```python
from build123d import *

# Parameters (mm, degrees)
BOSS_EXTRUDE1_DEPTH  = 12.5
BOSS_EXTRUDE2_DEPTH  = 3.4
BOSS_EXTRUDE3_DEPTH  = 3.5000000000000004
SKETCH4_W            = 0.40000000000000124
SKETCH4_H            = 6.935639852470931
CUT_EXTRUDE1_DEPTH   = 15.890601062415177
CUT_EXTRUDE2_DEPTH   = 18.660124574872064
BOSS_EXTRUDE4_DEPTH  = 0.29999999999999993
SKETCH7_W            = 1.7000000000000002
SKETCH7_H            = 9.6
BOSS_EXTRUDE5_DEPTH  = 0.5000000000000003
BOSS_EXTRUDE6_DEPTH  = 0.3
CUT_EXTRUDE3_DEPTH   = 15.890601062415183
SKETCH10_W           = 1.4499999999999997
SKETCH10_H           = 1
BOSS_EXTRUDE7_DEPTH  = 0.3
BOSS_EXTRUDE8_DEPTH  = 0.3
BOSS_EXTRUDE9_START  = 0.3
BOSS_EXTRUDE9_DEPTH  = 0.3
SKETCH13_W           = 3.3000000000000003
SKETCH13_H           = 0.3
CUT_EXTRUDE4_DEPTH   = 16.455824144962317
SKETCH14_W           = 3.3
SKETCH14_H           = 0.3
CUT_EXTRUDE5_DEPTH   = 1.7
SKETCH15_W           = 3.3
SKETCH15_H           = 0.3
CUT_EXTRUDE6_DEPTH   = 18.38620142526826
CUT_EXTRUDE7_REACH   = 19.386
SKETCH16_W           = 3.3
SKETCH16_H           = 0.3
BOSS_EXTRUDE10_DEPTH = 1.14
BOSS_EXTRUDE11_DEPTH = 1.14
BOSS_EXTRUDE12_DEPTH = 1.14
BOSS_EXTRUDE13_DEPTH = 1.14
CUT_EXTRUDE8_DEPTH   = 9.1
SKETCH22_W           = 1.1399999999999995
SKETCH22_H           = 1.1400000000000003
BOSS_EXTRUDE14_DEPTH = 5.6000000000000005
SKETCH23_W           = 3.5
SKETCH23_H           = 3.4999999999999996
CUT_EXTRUDE9_DEPTH   = 9.1
SKETCH24_W           = 1.14
SKETCH24_H           = 1.1400000000000003
BOSS_EXTRUDE15_DEPTH = 5.6000000000000005
CUT_EXTRUDE10_DEPTH  = 9.1
BOSS_EXTRUDE16_DEPTH = 5.6000000000000005
SKETCH27_W           = 3.5
SKETCH27_H           = 3.4999999999999996
CUT_EXTRUDE11_DEPTH  = 9.1
SKETCH28_W           = 1.1399999999999995
SKETCH28_H           = 1.1400000000000006
BOSS_EXTRUDE17_DEPTH = 5.6000000000000005
DRAFT1_ANGLE         = -5.000000000000134
DRAFT2_ANGLE         = 39.99999999999766
CHAMFER1_SIZE        = 1.0000000000000708
CHAMFER2_SIZE        = 0.7999999999999999
FILLET1_R            = 0.3


with BuildPart() as part:
    # Sketch1 → Boss-Extrude1 (new body)
    with BuildSketch(Plane.XZ.offset(-0.3)):
        with BuildLine():
            Line((-4.8, -4.8), (1.7000000000000002, -4.8))
            Line((1.7000000000000002, -4.8), (1.7000000000000002, 4.800000000000001))
            Line((1.7000000000000002, 4.800000000000001), (-4.8, 4.8))
            Line((-4.8, 4.8), (-4.8, -2.2))
            ThreePointArc((-4.8, -2.2), (-5.2, -2.6000000000000005), (-4.8, -3.0000000000000004))
            Line((-4.8, -3.0000000000000004), (-4.8, -4.8))
        make_face()
    extrude(amount=-BOSS_EXTRUDE1_DEPTH)

    # Sketch2 → Boss-Extrude2 (add)
    with BuildSketch(Plane(origin=(1.7, 0, 0), x_dir=(0, 0, -1), z_dir=(1, 0, 0))):
        Polygon((-4.800000000000008, 12.800000000000006), (-6.200000000000001, 10.45), (-6.200000000000001, 9.627515871063899), (-4.800000000000008, 9.627515871063899), align=None)
    extrude(amount=-BOSS_EXTRUDE2_DEPTH)

    # Sketch3 → Boss-Extrude3 (add)
    with BuildSketch(Plane(origin=(1.7000000000000002, 0, 0), x_dir=(0, 0, -1), z_dir=(1, 0, 0))):
        Polygon((4.8, 0.29999999999999993), (-4.800000000000001, 0.29999999999999993), (-4.8, 12.8), (4.8, 12.8), align=None)
    extrude(amount=BOSS_EXTRUDE3_DEPTH)

    # Sketch4 → Cut-Extrude1 (cut, through all)
    with BuildSketch(Plane(origin=(0, 12.8, 0), x_dir=(-1, 0, 0), z_dir=(0, 1, 0))):
        with Locations((-5, -1.3321800737645344)):
            Rectangle(SKETCH4_W, SKETCH4_H)
    extrude(amount=-CUT_EXTRUDE1_DEPTH, mode=Mode.SUBTRACT)

    # Sketch5 → Cut-Extrude2 (cut, through all)
    with BuildSketch(Plane(origin=(0, 0, -4.8), x_dir=(-1, 0, 0), z_dir=(0, 0, -1))):
        Polygon((-3.35, 0.29999999999999993), (3.3499999999999996, 0.29999999999999993), (3.35, 0.5000000000000001), (-3.35, 0.5000000000000004), align=None)
    extrude(amount=-CUT_EXTRUDE2_DEPTH, mode=Mode.SUBTRACT)

    # Sketch6 → Boss-Extrude4 (add)
    with BuildSketch(Plane.XZ.offset(-0.3)):
        Polygon((4.8, -4.8), (3.35, -4.8), (3.35, 0.49999999999999956), (4.8, 0.5), align=None)
    extrude(amount=BOSS_EXTRUDE4_DEPTH)

    # Sketch7 → Boss-Extrude5 (add)
    with BuildSketch(Plane.XZ.offset(-0.5000000000000002)):
        Rectangle(SKETCH7_W, SKETCH7_H)
    extrude(amount=BOSS_EXTRUDE5_DEPTH)

    # Sketch8 → Boss-Extrude6 (add)
    with BuildSketch(Plane.XZ.offset(-0.3)):
        Polygon((-4.8, -4.8), (-4.8, -3.8), (-3.3499999999999996, -3.8), (-3.35, -4.8), align=None)
    extrude(amount=BOSS_EXTRUDE6_DEPTH)

    # Sketch9 → Cut-Extrude3 (cut, through all)
    with BuildSketch(Plane.XZ.offset(-0.3)):
        Polygon((5.200000000000001, 4.800000000000001), (4.8, 4.800000000000001), (4.8, 3.464360147529), (5.200000000000001, 3.4643601475289993), align=None)
    extrude(amount=-CUT_EXTRUDE3_DEPTH, mode=Mode.SUBTRACT)

    # Sketch10 → Boss-Extrude7 (add)
    with BuildSketch(Plane.XZ.offset(-0.3)):
        with Locations((4.075, 4.3)):
            Rectangle(SKETCH10_W, SKETCH10_H)
    extrude(amount=BOSS_EXTRUDE7_DEPTH)

    # Sketch11 → Boss-Extrude8 (add)
    with BuildSketch(Plane.XZ.offset(-0.3)):
        Polygon((-4.8, 4.8), (-3.3499999999999996, 4.8), (-3.35, -0.49999999999999956), (-4.8, -0.5), align=None)
    extrude(amount=BOSS_EXTRUDE8_DEPTH)

    # Sketch12 → Boss-Extrude9 (add)
    with BuildSketch(Plane.XZ.offset(-0.3).offset(BOSS_EXTRUDE9_START)):
        with BuildLine():
            Line((-4.8, -2.2), (-4.8, -3.0000000000000004))
            ThreePointArc((-4.8, -3.0000000000000004), (-5.199999999999999, -2.6000000000000005), (-4.8, -2.2))
        make_face()
    extrude(amount=-BOSS_EXTRUDE9_DEPTH)

    # Sketch13 → Cut-Extrude4 (cut, through all)
    with BuildSketch(Plane.ZY.offset(0.8500000000000001)):
        with Locations((2.15, 0.15000000000000005)):
            Rectangle(SKETCH13_W, SKETCH13_H)
    extrude(amount=-CUT_EXTRUDE4_DEPTH, mode=Mode.SUBTRACT)

    # Sketch14 → Cut-Extrude5 (cut)
    with BuildSketch(Plane.ZY.offset(0.8500000000000001)):
        with Locations((-2.15, 0.15000000000000005)):
            Rectangle(SKETCH14_W, SKETCH14_H)
    extrude(amount=-CUT_EXTRUDE5_DEPTH, mode=Mode.SUBTRACT)

    # Sketch15 → Cut-Extrude6 (cut, through all)
    with BuildSketch(Plane.ZY.offset(4.8)):
        with Locations((2.15, 0.15)):
            Rectangle(SKETCH15_W, SKETCH15_H)
    extrude(amount=-CUT_EXTRUDE6_DEPTH, mode=Mode.SUBTRACT)

    # Sketch16 → Cut-Extrude7 (cut, up to next)
    with BuildSketch(Plane(origin=(4.8, 0, 0), x_dir=(0, 0, -1), z_dir=(1, 0, 0)), mode=Mode.PRIVATE) as cut_extrude7_sk1:
        with Locations((2.15, 0.15)):
            Rectangle(SKETCH16_W, SKETCH16_H)
    cut_extrude7_tool1 = extrude(cut_extrude7_sk1.sketch, amount=-CUT_EXTRUDE7_REACH, mode=Mode.PRIVATE) & part.part
    add(cut_extrude7_tool1.solids().sort_by_distance((4.8, 0.15, -2.15))[0], mode=Mode.SUBTRACT)

    # Sketch17 → Boss-Extrude10 (add)
    with BuildSketch(Plane(origin=(1.53, 0, 0), x_dir=(0, -1, 0), z_dir=(-1, 0, 0))):
        Polygon((2.500000000000003, 2.6499999999999937), (3.5, 3.085), (3.5, 3.2500000000000004), (-0.5, 3.2500000000000004), (-0.5, 2.6500000000000004), align=None)
    extrude(amount=-BOSS_EXTRUDE10_DEPTH)

    # Sketch18 → Boss-Extrude11 (add)
    with BuildSketch(Plane(origin=(1.53, 0, 0), x_dir=(0, -1, 0), z_dir=(-1, 0, 0))):
        Polygon((3.5, -2.85), (3.4999999999999987, -2.685000000000003), (2.5000000000000004, -2.2500000000000004), (-0.5, -2.2500000000000004), (-0.5, -2.85), align=None)
    extrude(amount=-BOSS_EXTRUDE11_DEPTH)

    # Sketch19 → Boss-Extrude12 (add)
    with BuildSketch(Plane(origin=(-2.6700000000000004, 0, 0), x_dir=(0, -1, 0), z_dir=(-1, 0, 0))):
        Polygon((2.500000000000003, 2.6499999999999937), (3.5, 3.085), (3.5, 3.2500000000000004), (-0.5, 3.2500000000000004), (-0.5, 2.6500000000000004), align=None)
    extrude(amount=-BOSS_EXTRUDE12_DEPTH)

    # Sketch20 → Boss-Extrude13 (add)
    with BuildSketch(Plane(origin=(-2.6700000000000004, 0, 0), x_dir=(0, -1, 0), z_dir=(-1, 0, 0))):
        Polygon((3.5, -2.85), (3.4999999999999987, -2.685000000000003), (2.5000000000000004, -2.2500000000000004), (-0.5, -2.2500000000000004), (-0.5, -2.85), align=None)
    extrude(amount=-BOSS_EXTRUDE13_DEPTH)

    # Sketch21 → Cut-Extrude8 (cut)
    with BuildSketch(Plane(origin=(0, 12.8, 0), x_dir=(-1, 0, 0), z_dir=(0, 1, 0))):
        Polygon((0.3499999999999999, 4.05), (0.34999999999999964, 0.5500000000000002), (3.85, 0.5500000000000002), (3.85, 4.05), align=None)
    extrude(amount=-CUT_EXTRUDE8_DEPTH, mode=Mode.SUBTRACT)

    # Sketch22 → Boss-Extrude14 (add)
    with BuildSketch(Plane(origin=(0, 3.7, 0), x_dir=(-1, 0, 0), z_dir=(0, 1, 0))):
        with Locations((2.0999999999999996, 2.3)):
            Rectangle(SKETCH22_W, SKETCH22_H)
    extrude(amount=BOSS_EXTRUDE14_DEPTH)

    # Sketch23 → Cut-Extrude9 (cut)
    with BuildSketch(Plane(origin=(0, 12.8, 0), x_dir=(-1, 0, 0), z_dir=(0, 1, 0))):
        with Locations((-2.1, 2.3)):
            Rectangle(SKETCH23_W, SKETCH23_H)
    extrude(amount=-CUT_EXTRUDE9_DEPTH, mode=Mode.SUBTRACT)

    # Sketch24 → Boss-Extrude15 (add)
    with BuildSketch(Plane(origin=(0, 3.7, 0), x_dir=(-1, 0, 0), z_dir=(0, 1, 0))):
        with Locations((-2.1, 2.3)):
            Rectangle(SKETCH24_W, SKETCH24_H)
    extrude(amount=BOSS_EXTRUDE15_DEPTH)

    # Sketch25 → Cut-Extrude10 (cut)
    with BuildSketch(Plane(origin=(0, 12.8, 0), x_dir=(-1, 0, 0), z_dir=(0, 1, 0))):
        Polygon((-3.85, -0.14999999999999997), (-3.85, -3.6499999999999995), (-0.3499999999999998, -3.6499999999999995), (-0.3499999999999999, -0.14999999999999997), align=None)
    extrude(amount=-CUT_EXTRUDE10_DEPTH, mode=Mode.SUBTRACT)

    # Sketch26 → Boss-Extrude16 (add)
    with BuildSketch(Plane(origin=(0, 3.7, 0), x_dir=(-1, 0, 0), z_dir=(0, 1, 0))):
        Polygon((-2.67, -2.4700000000000006), (-2.67, -1.3300000000000003), (-1.53, -1.33), (-1.53, -2.4700000000000006), align=None)
    extrude(amount=BOSS_EXTRUDE16_DEPTH)

    # Sketch27 → Cut-Extrude11 (cut)
    with BuildSketch(Plane(origin=(0, 12.8, 0), x_dir=(-1, 0, 0), z_dir=(0, 1, 0))):
        with Locations((2.1, -1.8999999999999997)):
            Rectangle(SKETCH27_W, SKETCH27_H)
    extrude(amount=-CUT_EXTRUDE11_DEPTH, mode=Mode.SUBTRACT)

    # Sketch28 → Boss-Extrude17 (add)
    with BuildSketch(Plane(origin=(0, 3.7, 0), x_dir=(-1, 0, 0), z_dir=(0, 1, 0))):
        with Locations((2.0999999999999996, -1.9000000000000004)):
            Rectangle(SKETCH28_W, SKETCH28_H)
    extrude(amount=BOSS_EXTRUDE17_DEPTH)

    # Draft1
    draft1_faces = [part.faces().sort_by_distance(p)[0] for p in [
        (-5e-17, 9.627515871063899, 5.500000000000004),
    ]]
    draft(draft1_faces, Plane(origin=(-1.7, 10.45, 6.200000000000001), x_dir=(1, 0, 0), z_dir=(0, 0, 1)), DRAFT1_ANGLE)

    # Draft2
    draft2_faces = [part.faces().sort_by_distance(p)[0] for p in [
        (5.000000000000001, 6.550000000000001, 3.4643601475290002),
        (5.000000000000001, 6.550000000000001, 2.135639852470931),
    ]]
    draft(draft2_faces, Plane(origin=(5.200000000000001, 0, 0), x_dir=(0, 0, 1), z_dir=(1, 0, 0)), DRAFT2_ANGLE)

    # Chamfer1
    chamfer1_edges = [part.edges().sort_by_distance(p)[0] for p in [
        (0.3499999999999998, 8.25, -3.6499999999999995),
        (3.85, 8.25, -3.6499999999999995),
    ]]
    chamfer(chamfer1_edges, length=CHAMFER1_SIZE)

    # Chamfer2
    chamfer2_edges = [part.edges().sort_by_distance(p)[0] for p in [
        (-3.85, 8.25, 0.5500000000000002),
        (-0.34999999999999964, 8.25, 0.5500000000000002),
    ]]
    chamfer(chamfer2_edges, length=CHAMFER2_SIZE)

    # Fillet1
    fillet1_edges = [part.edges().sort_by_distance(p)[0] for p in [
        (-4.8, 6.4, 4.8),
        (-4.8, 6.4, -4.8),
        (4.8, 6.4, 4.800000000000001),
        (4.8, 6.4, -4.8),
    ]]
    fillet(fillet1_edges, radius=FILLET1_R)


solid = part.part
```
Build history of the part. All positions in model axes, mm. A direction names the side the tool comes from. Give positions to 0.01 mm unless a question says otherwise; leave off trailing zeros. Loops run counter-clockwise (first coordinate to the right, second up) from the corner with the lowest first, then second, coordinate; pieces in that order, holes last.
1) 3-axis set-ups, long thin cutter, end or side, ignore diameter. For faces 1 (the face through (0.35, 8, 2)), 2 (the face through (-4.8, 6, 1)), 3 (the face through (-2.108, -2.993, 2.864)): which of +Z, -Z, +X, -X, +Y, -Y reach the whole face in a straight line?
Values follow:
face 1: +Y
face 2: +Z, -X, +Y, -Y
face 3: +X, -X, -Y
2) Drop flat-ended pins along their axis: P1, Ø1.2, axis at x = -4, z = -1.5, coming from the -Y side; P2, Ø1.7, axis at x = -2.5, z = 2.5, coming from the +Y side; P3, Ø2, axis at y = 7, z = 3, coming from the -X side. Give the stop position or say it passes through.
Values follow:
P1: stops at y = 0.3
P2: stops at y = 9.3
P3: stops at x = -4.8
3) Band-saw the part on D-D on y = 6. State how many separate pieces and enclosed holes the cut face has, then the cut area to 3 significant figures.
Values follow:
separate pieces: 5
enclosed holes: 4
area: 50.8 mm2
4) Band-saw the part on A-A on y = -2.25. List the corners of the cut face in (x, z).
Values follow:
outline: (-2.67, -2.85) - (-1.53, -2.85) - (-1.53, -2.25) - (-2.67, -2.25) - close; (-2.67, 2.65) - (-1.53, 2.65) - (-1.53, 3.25) - (-2.67, 3.25) - close; (1.53, -2.85) - (2.67, -2.85) - (2.67, -2.25) - (1.53, -2.25) - close; (1.53, 2.65) - (2.67, 2.65) - (2.67, 3.25) - (1.53, 3.25) - close
5) Band-saw the part on B-B on y = 0.75. List the corners of the cut face in (x, z), then the cut area to 3 significant figures.
Values follow:
outline: (-4.8, -4.5) arc R0.3 ccw to (-4.5, -4.8) - (4.5, -4.8) arc R0.3 ccw to (4.8, -4.5) - (4.8, 1.8) - (5.2, 2.14) - (5.2, 3.46) - (4.8, 3.8) - (4.8, 4.5) arc R0.3 ccw to (4.5, 4.8) - (-4.5, 4.8) arc R0.3 ccw to (-4.8, 4.5) - (-4.8, -2.2) arc R0.4 ccw to (-4.8, -3) - close
area: 93.0 mm2
6) Probe line 1 along X through (y, z) = (6.25, 1.5); line 2 along Z through (x, y) = (0, 0.25); line 3 along Z through (x, y) = (-3, 7.75). List the from-to ranges inside material, lowest first.
Values follow:
line 1: x = -4.8 to -3.85, -0.35 to 0.35, 3.85 to 4.8
line 2: z = -4.8 to -3.8, -0.5 to 0.5, 3.8 to 4.8
line 3: z = -4.8 to -3.65, -0.15 to 0.55, 4.05 to 4.8
